Verification items for the finished model (mm, model axes). A direction names the side the tool comes from. Coordinates: 2 decimals unless noted, no trailing zeros. Write each loop counter-clockwise with the first axis right and the second up, starting at its lowest first coordinate (ties: lowest second). Pieces come first, ordered by that corner, then holes. Notation, with made-up numbers: (-31, 10.25) -> (1, 10.25) arc R35 ccw to (1, 46.25) -> close; hole circle Ø10 at (-22.5, -32.5). An arc over 180 degrees is marked (long way). Answer in a Markdown table with one row per item.
```python
from build123d import *

# Parameters (mm, degrees)
EXTRUDE_THIN1_DEPTH = 152.4
CUT_EXTRUDE1_DEPTH  = 187.089943391
BOSS_EXTRUDE1_DEPTH = 101.6


with BuildPart() as part:
    # Sketch1 → Extrude-Thin1 (new body)
    with BuildSketch(Plane.XY):
        with BuildLine():
            ThreePointArc((0, -6.35), (3.175, -3.175), (0, 0))
            Line((0, 0), (-101.6, 0))
            ThreePointArc((-101.6, 0), (-104.775, -3.175), (-101.6, -6.35))
            Line((-101.6, -6.35), (-101.6, -7.9375))
            ThreePointArc((-101.6, -7.9375), (-106.3625, -3.175), (-101.6, 1.5875))
            Line((-101.6, 1.5875), (0, 1.5875))
            ThreePointArc((0, 1.5875), (4.7625, -3.175), (0, -7.9375))
            Line((0, -7.9375), (0, -6.35))
        make_face()
    extrude(amount=EXTRUDE_THIN1_DEPTH)

    # Sketch3 → Cut-Extrude1 (cut, through all)
    with BuildSketch(Plane(origin=(0, 1.5875, 0), x_dir=(1, 0, 0), z_dir=(0, 1, 0))):
        with BuildLine():
            Line((-53.975, -120.275242086), (-53.975, -28.949757914))
            ThreePointArc((-53.975, -28.949757914), (-50.8, -20.6375), (-47.625, -28.949757914))
            Line((-47.625, -28.949757914), (-47.625, -120.275242086))
            ThreePointArc((-47.625, -120.275242086), (-50.8, -128.5875), (-53.975, -120.275242086))
        make_face()
    extrude(amount=-CUT_EXTRUDE1_DEPTH, mode=Mode.SUBTRACT)

    # Sketch4 → Boss-Extrude1 (add)
    with BuildSketch(Plane(origin=(0, 0, 0), x_dir=(0, 0, -1), z_dir=(1, 0, 0))):
        with BuildLine():
            Line((-154.126058809, 0.997401867), (-190.844208608, -34.108402144))
            Line((-190.844208608, -34.108402144), (-189.747152233, -35.255844326))
            Line((-189.747152233, -35.255844326), (-153.029002434, -0.150040314))
            ThreePointArc((-153.029002434, -0.150040314), (-152.734811746, 0.010126107), (-152.4, 0))
            Line((-152.4, 0), (-152.4, 1.5875))
            ThreePointArc((-152.4, 1.5875), (-153.32800726, 1.482513557), (-154.126058809, 0.997401867))
        make_face()
    extrude(amount=-BOSS_EXTRUDE1_DEPTH)


solid = part.part
```
1. Mould release check, pull along Y, two halves, no side actions. Record for faces 4 (the cylindrical face through (-104.774, -3.105, 75.133)), 5 (the flat face through (-61, 0, 75)), 6 (the cylindrical face through (4.76, -3.07, 75.13)): released by +Y, released by -Y, zero draft, split by the parting line, or undercut.
Geometry says:
| item | result |
|---|---|
| face 4 | undercut |
| face 5 | released by -Y |
| face 6 | split by the parting line |
2. Thickness scan on line 1 (Y direction, x = -7, z = 149); line 2 (X direction, y = -4, z = 8); line 3 (X direction, y = -1, z = 122). Record the ranges inside material, lowest first. Write a range as from..to.
Geometry says:
| item | result |
|---|---|
| line 1 | 0..1.59 |
| line 2 | -106.29..-104.67, 3.07..4.69 |
| line 3 | -105.84..-103.91, 2.31..4.24 |
3. Depth check by flat-ended pin: P1, Ø1, axis at x = -57.5, y = -10, coming from the +Z side; P2, Ø0.8, axis at y = 1, z = 61, coming from the +X side; P3, Ø5, axis at x = -103, y = -1, coming from the +Z side; P4, Ø11, axis at y = -8, z = 175, coming from the -X side. Enter the tip coordinate at first touch or a pass-through.
Geometry says:
| item | result |
|---|---|
| P1 | z = 166.15 |
| P2 | x = 2.9 |
| P3 | z = 158.38 |
| P4 | through |
4. Section check B-B, the plane x = -6.5. Record the boundary of the cut face in (y, z).
Geometry says:
| item | result |
|---|---|
| outline | (-35.26, 189.75) -> (-0.15, 153.03) arc R0.64 cw to (0, 152.4) -> (0, 0) -> (1.59, 0) -> (1.59, 152.4) arc R2.17 ccw to (1, 154.13) -> (-34.11, 190.84) -> close |
5. Tool access check on faces 1 (the flat face through (-105, -3, 152.4)), 2 (the cylindrical face through (-106.36, -3.28, 75.13)), 3 (the flat face through (3.5, -3.1, 152.4)). Record the directions out of +Z, -Z, +X, -X, +Y, -Y that give a thin tool (end or side, any length) a straight path to the whole face; none if there is none.
Geometry says:
| item | result |
|---|---|
| face 1 | +Z, -X, +Y, -Y |
| face 2 | +Z, -Z, -X |
| face 3 | +Z, +X, +Y, -Y |
6. Section check D-D, the plane y = -29. Record the boundary of the cut face in (x, z), plus the area to 3 significant figures.
Geometry says:
| item | result |
|---|---|
| outline | (-101.6, 183.2) -> (0, 183.2) -> (0, 185.5) -> (-101.6, 185.5) -> close |
| area | 233 mm^2 |
